```python
from build123d import *

# Parameters (mm, degrees)
SKETCH1_W           = 71
SKETCH1_H           = 35
BOSS_EXTRUDE1_DEPTH = 2
SKETCH2_W           = 71
SKETCH2_H           = 35
SKETCH2_W_2         = 67
SKETCH2_H_2         = 31
BOSS_EXTRUDE2_DEPTH = 5
SKETCH3_W           = 52
SKETCH3_H           = 7
CUT_EXTRUDE1_DEPTH  = 5
SKETCH4_W           = 2
SKETCH4_H           = 31
SKETCH4_H_2         = 12
SKETCH4_H_3         = 6
BOSS_EXTRUDE3_DEPTH = 4
SKETCH5_W           = 13
SKETCH5_H           = 5
CUT_EXTRUDE2_DEPTH  = 2
SKETCH6_W           = 10
SKETCH6_H           = 5
CUT_EXTRUDE3_DEPTH  = 2
BOSS_EXTRUDE4_DEPTH = 1


with BuildPart() as part:
    # Sketch1 → Boss-Extrude1 (new body)
    with BuildSketch(Plane(origin=(0, 0, 0), x_dir=(1, 0, 0), z_dir=(0, 1, 0))):
        with Locations((35.5, 17.5)):
            Rectangle(SKETCH1_W, SKETCH1_H)
    extrude(amount=BOSS_EXTRUDE1_DEPTH)

    # Sketch2 → Boss-Extrude2 (add)
    with BuildSketch(Plane(origin=(0, 2, 0), x_dir=(1, 0, 0), z_dir=(0, 1, 0))):
        with Locations((35.5, 17.5)):
            Rectangle(SKETCH2_W, SKETCH2_H)
        with Locations((35.5, 17.5)):
            Rectangle(SKETCH2_W_2, SKETCH2_H_2, mode=Mode.SUBTRACT)
    extrude(amount=BOSS_EXTRUDE2_DEPTH)

    # Sketch3 → Cut-Extrude1 (cut)
    with BuildSketch(Plane(origin=(0, 2, 0), x_dir=(1, 0, 0), z_dir=(0, 1, 0))):
        with Locations((36, 29.5)):
            Rectangle(SKETCH3_W, SKETCH3_H)
    extrude(amount=-CUT_EXTRUDE1_DEPTH, mode=Mode.SUBTRACT)

    # Sketch4 → Boss-Extrude3 (add)
    with BuildSketch(Plane(origin=(0, 2, 0), x_dir=(1, 0, 0), z_dir=(0, 1, 0))):
        with Locations((3, 17.5)):
            Rectangle(SKETCH4_W, SKETCH4_H)
        with Locations((68, 27)):
            Rectangle(SKETCH4_W, SKETCH4_H_2)
        with Locations((68, 5)):
            Rectangle(SKETCH4_W, SKETCH4_H_3)
    extrude(amount=BOSS_EXTRUDE3_DEPTH)

    # Sketch5 → Cut-Extrude2 (cut)
    with BuildSketch(Plane.ZY.offset(-69)):
        with Locations((-14.5, 4.5)):
            Rectangle(SKETCH5_W, SKETCH5_H)
    extrude(amount=-CUT_EXTRUDE2_DEPTH, mode=Mode.SUBTRACT)

    # Sketch6 → Cut-Extrude3 (cut)
    with BuildSketch(Plane(origin=(0, 0, -2), x_dir=(-1, 0, 0), z_dir=(0, 0, -1))):
        with Locations((-46, 4.5)):
            Rectangle(SKETCH6_W, SKETCH6_H)
    extrude(amount=-CUT_EXTRUDE3_DEPTH, mode=Mode.SUBTRACT)

    # Sketch7 → Boss-Extrude4 (add)
    with BuildSketch(Plane(origin=(0, 7, 0), x_dir=(1, 0, 0), z_dir=(0, 1, 0))):
        Polygon((71, 35), (0, 35), (0, 0), (41, 0), (41, 1), (1, 1), (1, 34), (70, 34), (70, 21), (71, 21), align=None)
        Polygon((51, 0), (71, 0), (71, 8), (70, 8), (70, 1), (51, 1), align=None)
    extrude(amount=BOSS_EXTRUDE4_DEPTH)


solid = part.part
```
Design review of the part built by this model. Coordinates are the model's own, in mm. A direction names the side the tool comes from. Coordinates: 2 decimals unless noted, no trailing zeros. Loops run counter-clockwise (first coordinate to the right, second up) from the corner with the lowest first, then second, coordinate; pieces in that order, holes last.
Q1. We need section B-B on y = 4. State the section outline as (x, z) points.
Reported:
outline: (0, -35) - (71, -35) - (71, -21) - (67, -21) - (67, -33) - (4, -33) - (4, -2) - (41, -2) - (41, 0) - (0, 0) - close; (51, -2) - (67, -2) - (67, -8) - (71, -8) - (71, 0) - (51, 0) - close
Q2. For pin 1 (4 mm diameter, centred on x = 36.5, z = -23, fed in from +Y); pin 2 (1 mm diameter, centred on x = 68, z = -4.5, fed in from +Y), all flat-tipped, find the tip position at first contact; note any pin that passes through.
Reported:
pin 1: stops at y = 2
pin 2: stops at y = 6
Q3. The part is to be moulded in two halves that separate along X. For faces 5 (the face through (37, 2, -13)), 6 (the face through (71, 1, -17)), 7 (the face through (69, 4, -8)), say which applies: +X half, -X half, draft (parallel to the pull), parting line (faces both ways), or undercut.
Reported:
face 5: undercut
face 6: +X half
face 7: draft
Q4. Tool access review of faces 1 (the face through (67, 4, -27)), 2 (the face through (41, 5, -1)), 3 (the face through (69, 4, -21)), 4 (the face through (36, 1, -26)): name each direction out of +Z, -Z, +X, -X, +Y, -Y from which nothing blocks a thin tool from reaching the whole face with its end or side.
Reported:
face 1: +Y
face 2: +Z, +Y
face 3: +X, +Y
face 4: +Y, -Y
Q5. We need section D-D on y = 1. State the section outline as (x, z) points, and give its area (3 significant figures).
Reported:
outline: (0, -35) - (71, -35) - (71, 0) - (0, 0) - close; hole (10, -33) - (62, -33) - (62, -26) - (10, -26) - close
area: 2,120 mm2
Q6. We need section A-A on x = 47. State the section outline as (y, z) points, and give its area (3 significant figures).
Reported:
outline: (0, -35) - (8, -35) - (8, -34) - (7, -34) - (7, -33) - (0, -33) - close; (0, -26) - (2, -26) - (2, 0) - (0, 0) - close
area: 67.0 mm2
Q7. We need section C-C on z = -31.5. State the section outline as (x, y) points, and give its area (3 significant figures).
Reported:
outline: (0, 0) - (10, 0) - (10, 2) - (4, 2) - (4, 6) - (2, 6) - (2, 7) - (1, 7) - (1, 8) - (0, 8) - close; (62, 0) - (71, 0) - (71, 8) - (70, 8) - (70, 7) - (69, 7) - (69, 6) - (67, 6) - (67, 2) - (62, 2) - close
area: 76.0 mm2
Q8. To check wall thickness, follow line 1 (Z direction, x = 28.5, y = 5.5); line 2 (X direction, y = 7.75, z = -32.5); line 3 (X direction, y = 4.25, z = -29.5). State the ranges of each line that lie inside material, in increasing order.
Reported:
line 1: z = -35 to -33, -2 to 0
line 2: x = 0 to 1, 70 to 71
line 3: x = 0 to 4, 67 to 71
